```python
from build123d import *

# Parameters (mm, degrees)
BODY_DEPTH                      = 0.9
SIDE_EXTENDER_2_R               = 1.75
SIDE_EXTENDER_DEPTH             = 1.8
CENTER_EXTERN_W                 = 3
CENTER_EXTERN_H                 = 13.8
EXTENDER_CENTER_DEPTH           = 1.8
HOLES_R                         = 1.1
HOLES_R_2                       = 0.6
SCREW_HOLES_DEPTH               = 1.8
SHAFT_HOLE_R                    = 2.4
MOTOR_SHAFT_DEPTH               = 1.8
SKIZZE6_R                       = 1
SKIZZE6_R_2                     = 1.45
SCHNITT_LINEAR_AUSTRAGEN5_DEPTH = 0.8
VERRUNDUNG1_R                   = 1
VERRUNDUNG2_R                   = 0.5


with BuildPart() as part:
    # body 2 → body (new body, symmetric)
    with BuildSketch(Plane.XY):
        Polygon((0, 16.193693694), (-2.8, 16.193693694), (-2.8, 14.493693694), (-5.6, 14.493693694), (-5.6, 0.693693694), (-2.8, 0.693693694), (-2.8, -1.006306306), (0, -1.006306306), (2.8, -1.006306306), (2.8, 0.693693694), (5.6, 0.693693694), (5.6, 14.493693694), (2.8, 14.493693694), (2.8, 16.193693694), align=None)
    extrude(amount=BODY_DEPTH, both=True)

    # side_extender 2 → side-extender (add)
    with BuildSketch(Plane.XY.offset(0.9)):
        with Locations((0, 15.667972906)):
            Circle(SIDE_EXTENDER_2_R)
        with Locations((-0.0089251, -0.332027094)):
            Circle(SIDE_EXTENDER_2_R)
    extrude(amount=-SIDE_EXTENDER_DEPTH)

    # center-extern → Extender-center (add)
    with BuildSketch(Plane.XY.offset(0.9)):
        with BuildLine():
            Line((-5.6, 11.043693694), (-5.6, 4.143693694))
            ThreePointArc((-5.6, 4.143693694), (-9.05, 7.593693694), (-5.6, 11.043693694))
        make_face()
        with Locations((5.6, 7.593693694)):
            Rectangle(CENTER_EXTERN_W, CENTER_EXTERN_H)
    extrude(amount=-EXTENDER_CENTER_DEPTH)

    # holes → screw-holes (cut)
    with BuildSketch(Plane.XY.offset(0.9)):
        with Locations((-7.154497296, 7.593693694)):
            Circle(HOLES_R)
        with Locations((-0.000834968, 15.593693694)):
            Circle(HOLES_R)
        with Locations((-0.008158127, -0.406306306)):
            Circle(HOLES_R)
        with Locations((-0.002436909, 12.093693694)):
            Circle(HOLES_R_2)
        with Locations((-0.006556186, 3.093693694)):
            Circle(HOLES_R_2)
    extrude(amount=-SCREW_HOLES_DEPTH, mode=Mode.SUBTRACT)

    # shaft hole → motor shaft (cut)
    with BuildSketch(Plane.XY.offset(0.9)):
        with Locations((-0.00446255, 7.603703107)):
            Circle(SHAFT_HOLE_R)
    extrude(amount=-MOTOR_SHAFT_DEPTH, mode=Mode.SUBTRACT)

    # Skizze6 → Schnitt-Linear austragen5 (cut)
    with BuildSketch(Plane.XY.offset(0.9)):
        with Locations((-0.002436909, 12.093693694)):
            Circle(SKIZZE6_R)
        with Locations((-0.006556186, 3.093693694)):
            Circle(SKIZZE6_R)
        with Locations((-0.000834968, 15.593693694)):
            Circle(SKIZZE6_R_2)
        with Locations((-0.008158127, -0.406306306)):
            Circle(SKIZZE6_R_2)
        with Locations((-7.154497296, 7.593693694)):
            Circle(SKIZZE6_R_2)
    extrude(amount=-SCHNITT_LINEAR_AUSTRAGEN5_DEPTH, mode=Mode.SUBTRACT)

    # Verrundung1
    verrundung1_edges = [part.edges().sort_by_distance(p)[0] for p in [
        (-5.6, 0.693693694, 0),
        (-5.6, 14.493693694, 0),
        (7.1, 0.693693694, 0),
        (7.1, 14.493693694, 0),
    ]]
    fillet(verrundung1_edges, radius=VERRUNDUNG1_R)

    # Verrundung2
    verrundung2_edges = [part.edges().sort_by_distance(p)[0] for p in [
        (2.8, 16.193693694, 0),
        (2.8, -1.006306306, 0),
        (-2.8, -1.006306306, 0),
        (-2.8, 16.193693694, 0),
    ]]
    fillet(verrundung2_edges, radius=VERRUNDUNG2_R)


solid = part.part
```
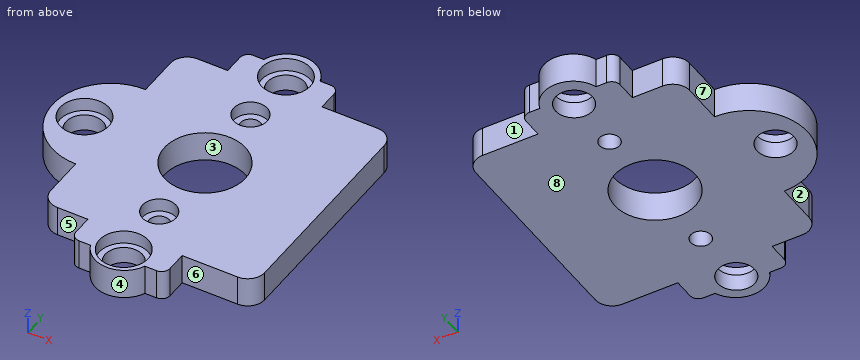
Here's how the part is built. I have some questions about the finished solid (model axes, mm). Face numbers are marked on the shaded views. A direction names the side the tool comes from. Give positions to 0.01 mm unless a question says otherwise; leave off trailing zeros. Write each loop counter-clockwise with the first axis right and the second up, starting at its lowest first coordinate (ties: lowest second). Pieces come first, ordered by that corner, then holes.
(1) Thinking about a two-plate mould opening in Y: for the marked faces 1, 2, 3 and 4, which applies, pulls with the +Y half, pulls with the -Y half, needs draft (parallel to the pull), parting line crosses it, or undercut?
Output values:
face 1: pulls with the +Y half
face 2: needs draft
face 3: undercut
face 4: pulls with the -Y half
(2) Imagine slicing it at A-A, the plane x = -7.5. Write out the boundary of the cut face in (y, z).
Output values:
outline: (4.71, -0.9) - (6.55, -0.9) - (6.55, 0.1) - (6.19, 0.1) - (6.19, 0.9) - (4.71, 0.9) - close; (8.64, -0.9) - (10.47, -0.9) - (10.47, 0.9) - (9, 0.9) - (9, 0.1) - (8.64, 0.1) - close
(3) Imagine slicing it at B-B, the plane z = -0.25. Count the separate pieces of the cut face and the enclosed holes in it, and give its area (3 significant figures).
Output values:
separate pieces: 1
enclosed holes: 6
area: 186 mm2
(4) Imagine slicing it at C-C, the plane y = 0. Write out the boundary of the cut face in (x, z), and give its area (3 significant figures).
Output values:
outline: (-2.8, -0.9) - (-1.03, -0.9) - (-1.03, 0.1) - (-1.4, 0.1) - (-1.4, 0.9) - (-2.8, 0.9) - close; (1.01, -0.9) - (2.8, -0.9) - (2.8, 0.9) - (1.38, 0.9) - (1.38, 0.1) - (1.01, 0.1) - close
area: 5.81 mm2
(5) Will these pins go through, and if not, where does the flat tip stop? pin 1 (0.5 mm diameter, centred on x = -3.5, z = -0.5, fed in from +Y); pin 2 (0.5 mm diameter, centred on y = 12, z = 0.5, fed in from -X); pin 3 (2 mm diameter, centred on x = 0, y = 15.59, fed in from -Z); pin 4 (1 mm diameter, centred on x = 0, y = 3.5, fed in from +Z).
Output values:
pin 1: stops at y = 14.49
pin 2: stops at x = -5.6
pin 3: passes through
pin 4: stops at z = 0.1
(6) On a 3-axis mill with a long thin cutter (end or side, diameter ignored), from which of +Z, -Z, +X, -X, +Y, -Y can I reach the whole of each face in a straight line? I mean the marked faces 5, 6, 7 and 8. Say none if no direction works.
Output values:
face 5: +Z, -Z, -X, -Y
face 6: +Z, -Z, +X, -Y
face 7: +Z, -Z, -X, +Y
face 8: -Z, +X, -X, +Y, -Y
(7) If I drill on L1, parallel to Y at x = 0, z = -0.6; L2, parallel to X at y = -0.5, z = -0.7; L3, parallel to X at y = 8, z = 0.55, over which ranges is the centre line in solid material (lowest first)?
Output values:
L1: y = -2.08 to -1.51, 0.69 to 2.49, 3.69 to 5.2, 10 to 11.49, 12.69 to 14.49, 16.69 to 17.42
L2: x = -2.8 to -1.1, 1.09 to 2.8
L3: x = -9.03 to -8.55, -5.76 to -2.37, 2.36 to 7.1
(8) Imagine slicing it at D-D, the plane x = 5. Write out the boundary of the cut face in (y, z).
Output values:
outline: (0.69, -0.9) - (14.49, -0.9) - (14.49, 0.9) - (0.69, 0.9) - close
